Read the model definition and answer for the solid it produces. Units are mm, in the model's axes. Face numbers are marked on the shaded views. A direction names the side the tool comes from. Give positions to 0.01 mm unless a question says otherwise; leave off trailing zeros. Loops run counter-clockwise (first coordinate to the right, second up) from the corner with the lowest first, then second, coordinate; pieces in that order, holes last. Notation, with made-up numbers: (46, 84.25) -> (89, 84.25) arc R18 ccw to (89, 98.25) -> close; hole circle Ø10 at (-29, 75.25). An arc over 180 degrees is marked (long way). Return JSON: item names as keys, results as strings. Group by question number.
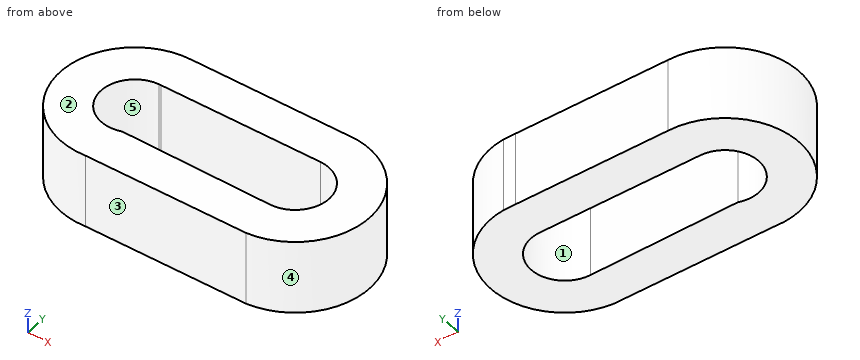
from build123d import *

# Parameters (mm, degrees)
F1_DEPTH = 17.4625


with BuildPart() as f1:
    # F0 (on Top) → F1 (new body)
    with BuildSketch(Plane.XY):
        with BuildLine():
            Line((-8.828322, -39.820505), (26.439151, -39.820505))
            Line((26.439151, -39.820505), (29.271678, -39.820505))
            ThreePointArc((29.271678, -39.820505), (45.317915, -22.415531), (29.271678, -5.010558))
            Line((29.271678, -5.010558), (26.487026, -5.006728))
            Line((26.487026, -5.006728), (-9.886203, -4.956709))
            ThreePointArc((-9.886203, -4.956709), (-27.699052, -22.945157), (-8.828322, -39.820505))
        make_face()
        with BuildLine():
            ThreePointArc((27.854786, -14.478031), (35.792759, -22.465207), (27.755437, -30.352402))
            Line((27.755437, -30.352402), (-7.620645, -29.906783))
            ThreePointArc((-7.620645, -29.906783), (-18.050575, -23.854432), (-10.464113, -14.481068))
            ThreePointArc((-10.464113, -14.481068), (-10.245214, -14.478031), (-10.026315, -14.481033))
            Line((-10.026315, -14.481033), (27.854786, -14.478031))
        make_face(mode=Mode.SUBTRACT)
    extrude(amount=F1_DEPTH)


solid = f1.part
1. Section C-C on x = -15 is taken. Determine the outline of the cut face in (y, z), then the cut area to 3 significant figures.
2. Section B-B on y = -23 is taken. Determine the outline of the cut face in (x, z).
3. Section D-D on y = -33 is taken. Determine the outline of the cut face in (x, z).
4. Which of the six approach directions +Z, -Z, +X, -X, +Y, -Y give full straight-line access (tool end or side, diameter ignored) to the marked faces 1 and 2?
5. Determine the mould class of the marked faces 3, 4 and 5 for opening direction X: pulls with the +X half, pulls with the -X half, needs draft (parallel to the pull), parting line crosses it, or undercut.
6. Section A-A on z = 15 is taken. Determine the outline of the cut face in (x, y) (1 decimal), then the cut area to 3 significant figures.
7. Straight lines are drawn through the part: line 1 (X direction, y = -22.5, z = 16.25); line 2 (Y direction, x = 26.5, z = 2); line 3 (Y direction, x = -6.5, z = 7.25). For each, find the intervals that lie inside material, in ascending order. Write a range as from..to.
8. Flat-ended cylindrical pins translate along their axes: pin 1 Ø1 at (y, z) = (-36, 6.5) entering from -X; pin 2 Ø5 at (x, z) = (0.5, 6.5) entering from -Y; pin 3 Ø10 at (y, z) = (-15, 15.5) entering from +X. Find the tip coordinate at first contact, or state that the pin passes through.
Completed:
{
 "1": {"outline": "(-39.22, 0) -> (-28.77, 0) -> (-28.77, 17.46) -> (-39.22, 17.46) -> close; (-16.06, 0) -> (-5.61, 0) -> (-5.61, 17.46) -> (-16.06, 17.46) -> close", "area": "365 mm²"},
 "2": {"outline": "(-27.7, 0) -> (-18.16, 0) -> (-18.16, 17.46) -> (-27.7, 17.46) -> close; (35.77, 0) -> (45.31, 0) -> (45.31, 17.46) -> (35.77, 17.46) -> close"},
 "3": {"outline": "(-24.13, 0) -> (41.74, 0) -> (41.74, 17.46) -> (-24.13, 17.46) -> close"},
 "4": {"face 1": "+Z, -Z", "face 2": "+Z, +X, -X, +Y, -Y"},
 "5": {"face 3": "needs draft", "face 4": "pulls with the +X half", "face 5": "undercut"},
 "6": {"outline": "(-9.9, -5) arc R17.5 ccw (long way) to (-8.8, -39.8) -> (29.3, -39.8) arc R17.5 ccw to (29.3, -5) -> (26.5, -5) -> close; hole (-10.5, -14.5) arc R7.9 ccw (long way) to (-7.6, -29.9) -> (27.8, -30.4) arc R7.9 ccw (long way) to (27.9, -14.5) -> (-10, -14.5) arc R7.9 ccw to start", "area": "1,490 mm²"},
 "7": {"line 1": "x = -27.71..-18.18, 35.79..45.32", "line 2": "y = -39.82..-30.34, -14.48..-5.01", "line 3": "y = -39.82..-29.92, -14.48..-4.96"},
 "8": {"pin 1": "stops at x = -21.81", "pin 2": "stops at y = -39.82", "pin 3": "stops at x = 45.15"}
}
